Build history of the part. All positions in model axes, mm. Face numbers are marked on the shaded views. Round coordinates to 2 decimals unless told otherwise and drop trailing zeros. Loops run counter-clockwise (first coordinate to the right, second up) from the corner with the lowest first, then second, coordinate; pieces in that order, holes last.
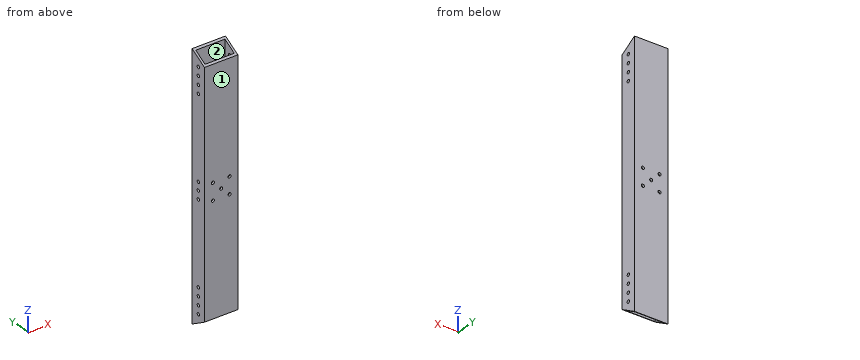
from build123d import *

# Parameters (mm, degrees)
SKETCH1_W           = 50.8
SKETCH1_H           = 25.4
SKETCH1_W_2         = 44.45
SKETCH1_H_2         = 19.05
BOSS_EXTRUDE1_DEPTH = 391.786872
CUT_EXTRUDE1_DEPTH  = 457.2
SKETCH3_R           = 2.38125
CUT_EXTRUDE2_DEPTH  = 394.430137472
SKETCH4_R           = 2.38125
CUT_EXTRUDE3_DEPTH  = 3.175
SKETCH5_R           = 2.38125
CUT_EXTRUDE4_DEPTH  = 396.270645345


with BuildPart() as part:
    # Sketch1 → Boss-Extrude1 (new body)
    with BuildSketch(Plane.XY):
        Rectangle(SKETCH1_W, SKETCH1_H)
        Rectangle(SKETCH1_W_2, SKETCH1_H_2, mode=Mode.SUBTRACT)
    extrude(amount=BOSS_EXTRUDE1_DEPTH)

    # Sketch2 → Cut-Extrude1 (cut)
    with BuildSketch(Plane(origin=(25.4, 0, 0), x_dir=(0, 0, -1), z_dir=(1, 0, 0))):
        Polygon((0, 12.7), (-14.664696837, -12.7), (0, -12.7), align=None)
        Polygon((-391.786872, -12.7), (-391.786872, 12.7), (-377.122175163, -12.7), align=None)
    extrude(amount=-CUT_EXTRUDE1_DEPTH, mode=Mode.SUBTRACT)

    # Sketch3 → Cut-Extrude2 (cut, through all)
    with BuildSketch(Plane(origin=(0, -12.7, 0), x_dir=(-1, 0, 0), z_dir=(0, -1, 0))):
        with Locations(Location((0, -195.893436, 0), (0, 0, 90))):
            Circle(SKETCH3_R)
        with Locations(Location((-12.7, -208.593436, 0), (0, 0, 90))):
            Circle(SKETCH3_R)
        with Locations(Location((12.7, -208.593436, 0), (0, 0, 90))):
            Circle(SKETCH3_R)
        with Locations(Location((-12.7, -183.193436, 0), (0, 0, 90))):
            Circle(SKETCH3_R)
        with Locations(Location((12.7, -183.193436, 0), (0, 0, 90))):
            Circle(SKETCH3_R)
    extrude(amount=-CUT_EXTRUDE2_DEPTH, mode=Mode.SUBTRACT)

    # Sketch4 → Cut-Extrude3 (cut)
    with BuildSketch(Plane.ZY.offset(25.4)):
        with Locations((195.893436, 0)):
            Circle(SKETCH4_R)
        with Locations((208.593436, 0)):
            Circle(SKETCH4_R)
        with Locations(Location((183.193436, 0, 0), (0, 0, 180))):
            Circle(SKETCH4_R)
    extrude(amount=-CUT_EXTRUDE3_DEPTH, mode=Mode.SUBTRACT)

    # Sketch5 → Cut-Extrude4 (cut, through all)
    with BuildSketch(Plane(origin=(25.4, 0, 0), x_dir=(0, 0, -1), z_dir=(1, 0, 0))):
        with Locations((-371.754523581, 0)):
            Circle(SKETCH5_R)
        with Locations((-359.054523581, 0)):
            Circle(SKETCH5_R)
        with Locations((-346.354523581, 0)):
            Circle(SKETCH5_R)
        with Locations((-333.654523581, 0)):
            Circle(SKETCH5_R)
        with Locations(Location((-58.132348419, 0, 0), (0, 0, 270))):
            Circle(SKETCH5_R)
        with Locations(Location((-45.432348419, 0, 0), (0, 0, 270))):
            Circle(SKETCH5_R)
        with Locations(Location((-32.732348419, 0, 0), (0, 0, 270))):
            Circle(SKETCH5_R)
        with Locations(Location((-20.032348419, 0, 0), (0, 0, 270))):
            Circle(SKETCH5_R)
    extrude(amount=-CUT_EXTRUDE4_DEPTH, mode=Mode.SUBTRACT)


solid = part.part
(1) Pull direction X, two halves, no side cores. Call the marked faces 1 and 2: +X half, -X half, draft (parallel to the pull), parting line (faces both ways), or undercut.
Responses:
face 1: draft
face 2: undercut
(2) Probe line 1 (Y direction, x = 4, z = 204.5) (3 decimals); line 2 (X direction, y = 8, z = 78.5) (3 decimals); line 3 (X direction, y = 2.25, z = 196.5) (3 decimals). List the from-to ranges inside material, lowest first.
Responses:
line 1: y = -12.7 to -9.525, 9.525 to 12.7
line 2: x = -25.4 to -22.225, 22.225 to 25.4
line 3: x = 22.225 to 25.4
(3) Pin check, flat tip, straight feed: P1, Ø4, axis at x = -12.7, z = 183.19, coming from the +Y side. Stop position of the tip, or through.
Responses:
P1: passes through
(4) Slice it at A-A on z = 39.5. List the corners of the cut face in (x, y) (3 decimals), plus the area to 3 significant figures.
Responses:
outline: (-25.4, -12.7) - (25.4, -12.7) - (25.4, 12.7) - (-25.4, 12.7) - close; hole (-22.225, -9.525) - (22.225, -9.525) - (22.225, 9.525) - (-22.225, 9.525) - close
area: 444 mm2
